For this review, use the dimensioned drawing (mm, ordinates from the lowest corner) and the shaded views. Give positions to 0.01 mm unless a question says otherwise; leave off trailing zeros. Write each loop counter-clockwise with the first axis right and the second up, starting at its lowest first coordinate (ties: lowest second). Pieces come first, ordered by that corner, then holes. Notation, with made-up numbers: M -4.75,20.25 L 32.25,20.25 A19 ccw 32.25,27.25 Z; hole C 76.25,69.25 d4. An arc over 180 degrees is marked long. Write each question's results on one line, items separated by ' | '. Start each with the question number.
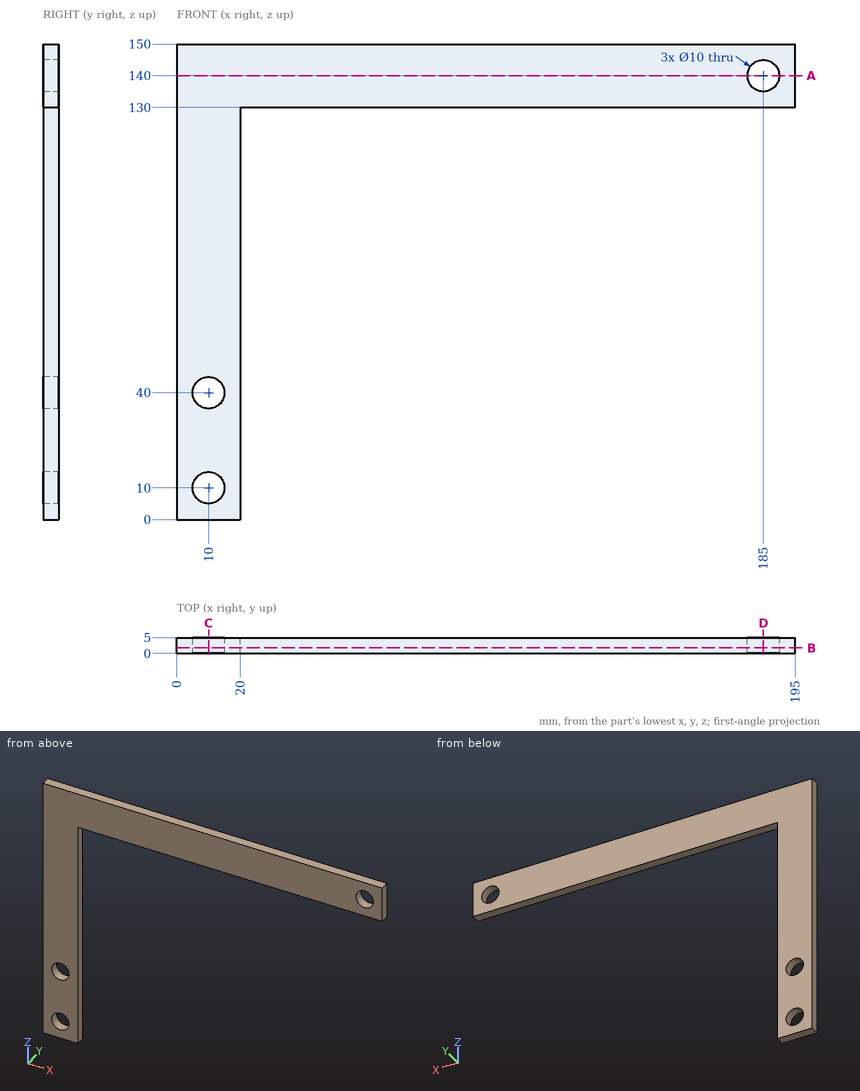
(1) Add section C-C (x = 10). State the section outline as (y, z) points, then the cut area to 3 significant figures.
(2) Add section A-A (z = 140). State the section outline as (x, y) points, then the cut area to 3 significant figures.
(3) Add section B-B (y = 1.75). State the section outline as (x, z) points, then the cut area to 3 significant figures.
(4) Wall thickness on L1, parallel to Z at x = 10, y = 1.7; L2, parallel to Z at x = 185, y = 2.95; L3, parallel to Z at x = 13, y = 0.2: over which ranges is each line inside the solid? List them lowest first.
(5) Clearance check with flat-ended pins moving along their axes: P1, Ø6, axis at x = 10, z = 40, coming from the -Y side; P2, Ø2.5, axis at x = 67, y = 3.5, coming from the -Z side; P3, Ø2.5, axis at y = 3.5, z = 89.5, coming from the +X side. State where each tip first meets the part, or that it passes through.
(6) Add section D-D (x = 185). State the section outline as (y, z) points, then the cut area to 3 significant figures.
Calculated:
1) outline: M 0,0 L 5,0 L 5,5 L 0,5 Z; M 0,15 L 5,15 L 5,35 L 0,35 Z; M 0,45 L 5,45 L 5,150 L 0,150 Z | area: 650 mm²
2) outline: M 0,0 L 180,0 L 180,5 L 0,5 Z; M 190,0 L 195,0 L 195,5 L 190,5 Z | area: 925 mm²
3) outline: M 0,0 L 20,0 L 20,130 L 195,130 L 195,150 L 0,150 Z; hole C 10,10 d10; hole C 10,40 d10; hole C 185,140 d10 | area: 6,260 mm²
4) L1: z = 0 to 5, 15 to 35, 45 to 150 | L2: z = 130 to 135, 145 to 150 | L3: z = 0 to 6, 14 to 36, 44 to 150
5) P1: passes through | P2: stops at z = 130 | P3: stops at x = 20
6) outline: M 0,130 L 5,130 L 5,135 L 0,135 Z; M 0,145 L 5,145 L 5,150 L 0,150 Z | area: 50.0 mm²
